from build123d import *

# Parameters (mm, degrees)
F0_R     = 0.6
F1_DEPTH = 1.7
F3_DEPTH = 2
F5_DEPTH = 1
F6_R     = 1.1
F7_DEPTH = 2.701
F8_R     = 2.35
F8_R_2   = 1.1
F9_DEPTH = 2


with BuildPart() as f1:
    # F0 (on Top) → F1 (new body)
    with BuildSketch(Plane.XY):
        with BuildLine():
            ThreePointArc((2.2299103121, -2.5), (3.057180036, -1.369726333), (3.35, 0))
            ThreePointArc((3.35, 0), (3.057180036, 1.369726333), (2.2299103121, 2.5))
            ThreePointArc((2.2299103121, 2.5), (0, 3.35), (-2.2299103121, 2.5))
            ThreePointArc((-2.2299103121, 2.5), (-3.35, 0), (-2.2299103121, -2.5))
            ThreePointArc((-2.2299103121, -2.5), (0, -3.35), (2.2299103121, -2.5))
        make_face()
        with BuildLine():
            ThreePointArc((2.2299103121, 2.5), (3.057180036, 1.369726333), (3.35, 0))
            ThreePointArc((3.35, 0), (3.057180036, -1.369726333), (2.2299103121, -2.5))
            Line((2.2299103121, -2.5), (14, -2))
            ThreePointArc((14, -2), (16, 0), (14, 2))
            Line((14, 2), (2.2299103121, 2.5))
        make_face()
        with Locations((4, 0)):
            Circle(F0_R, mode=Mode.SUBTRACT)
        with Locations((6, 0)):
            Circle(F0_R, mode=Mode.SUBTRACT)
        with Locations((8, 0)):
            Circle(F0_R, mode=Mode.SUBTRACT)
        with Locations((10, 0)):
            Circle(F0_R, mode=Mode.SUBTRACT)
        with Locations((12, 0)):
            Circle(F0_R, mode=Mode.SUBTRACT)
        with Locations((14, 0)):
            Circle(F0_R, mode=Mode.SUBTRACT)
        with BuildLine():
            ThreePointArc((-2.2299103121, -2.5), (-3.35, 0), (-2.2299103121, 2.5))
            Line((-2.2299103121, 2.5), (-9.1662129992, 2.2053419782))
            Line((-9.1662129992, 2.2053419782), (-9.1662129992, -2.2053419782))
            Line((-9.1662129992, -2.2053419782), (-2.2299103121, -2.5))
        make_face()
        with Locations((-8, 0)):
            Circle(F0_R, mode=Mode.SUBTRACT)
        with Locations((-6, 0)):
            Circle(F0_R, mode=Mode.SUBTRACT)
        with Locations((-4, 0)):
            Circle(F0_R, mode=Mode.SUBTRACT)
    extrude(amount=F1_DEPTH)

    # F2 (on face) → F3 (join)
    with BuildSketch(Plane.XY.offset(1.7)):
        with BuildLine():
            ThreePointArc((2.2299103121, -2.5), (3.057180036, -1.369726333), (3.35, 0))
            ThreePointArc((3.35, 0), (3.057180036, 1.369726333), (2.2299103121, 2.5))
            ThreePointArc((2.2299103121, 2.5), (0, 3.35), (-2.2299103121, 2.5))
            ThreePointArc((-2.2299103121, 2.5), (-3.35, 0), (-2.2299103121, -2.5))
            ThreePointArc((-2.2299103121, -2.5), (0, -3.35), (2.2299103121, -2.5))
        make_face()
    extrude(amount=F3_DEPTH)

    # F4 (on face) → F5 (cut)
    with BuildSketch(Plane(origin=(0, 0, 0), x_dir=(1, 0, 0), z_dir=(0, 0, -1))):
        with BuildLine():
            ThreePointArc((1.5642654428, 1.7537313433), (-2.35, 0), (1.5642654428, -1.7537313433))
            ThreePointArc((1.5642654428, -1.7537313433), (2.35, 0), (1.5642654428, 1.7537313433))
        make_face()
    extrude(amount=-F5_DEPTH, mode=Mode.SUBTRACT)

    # F6 (on face) → F7 (cut, through all)
    with BuildSketch(Plane(origin=(0, 0, 1), x_dir=(1, 0, 0), z_dir=(0, 0, -1))):
        Circle(F6_R)
    extrude(amount=-F7_DEPTH, mode=Mode.SUBTRACT)

    # F8 (on face) → F9 (cut, through all)
    with BuildSketch(Plane.XY.offset(3.7)):
        Circle(F8_R)
        Circle(F8_R_2, mode=Mode.SUBTRACT)
    extrude(amount=-F9_DEPTH, mode=Mode.SUBTRACT)


solid = f1.part
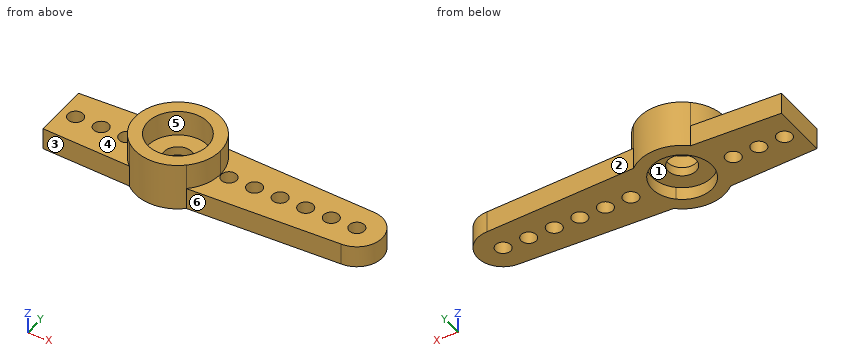
CAD build for the part. Positions are in the model's coordinates, mm. Face numbers are marked on the shaded views. A direction names the side the tool comes from. Give positions to 0.01 mm unless a question says otherwise; leave off trailing zeros. Loops run counter-clockwise (first coordinate to the right, second up) from the corner with the lowest first, then second, coordinate; pieces in that order, holes last. Notation, with made-up numbers: M -28.5,-17.5 L 28.5,-17.5 A36 ccw 28.5,20.5 Z; hole C 67,1.5 d11. An arc over 180 degrees is marked long. Answer in a Markdown table with one row per item. Add a question column.
Item 1: Band-saw the part on A-A on z = 1.4. Give the number of separate pieces and of enclosed holes in the cut face, then the cut area to 3 significant figures.
Item 2: Probe probe 1 along Y at (x, z) = (0, 3.1); probe 2 along Y at (x, z) = (14, 1.3); probe 3 along X at (y, z) = (-2, 2.6). List the from-to ranges inside material, lowest first.
Item 3: Band-saw the part on C-C on z = 3. Give the cut face in (x, y), then the cut area to 3 significant figures.
Item 4: Mould opens along X. For the marked faces 1, 2, 3 and 4 say: +X half, -X half, draft (parallel to the pull), parting line (faces both ways), or undercut.
Item 5: Band-saw the part on D-D on y = -1.5. Give the cut face in (x, z), then the cut area to 3 significant figures.
Item 6: Drop flat-ended pins along their axis: P1, Ø2.5, axis at x = 0, y = 0, coming from the -Z side; P2, Ø0.7, axis at x = 14, y = 0, coming from the -Z side; P3, Ø2, axis at y = -2, z = 2, coming from the -X side; P4, Ø1.4, axis at x = 12, y = 0, coming from the +Z side. Give the stop position or say it passes through.
Item 7: Band-saw the part on B-B on x = 8. Give the cut face in (y, z), then the cut area to 3 significant figures.
Item 8: Tool access for the marked faces 5 and 6: list every direction of +Z, -Z, +X, -X, +Y, -Y with a clear straight run to the whole face (end or side of a thin tool).
Reply:
| question | item | result |
|---|---|---|
| 1 | separate pieces | 1 |
| 1 | enclosed holes | 10 |
| 1 | area | 105 mm^2 |
| 2 | probe 1 | y = -3.35 to -2.35, 2.35 to 3.35 |
| 2 | probe 2 | y = -2 to -0.6, 0.6 to 2 |
| 2 | probe 3 | x = -2.69 to -1.23, 1.23 to 2.69 |
| 3 | outline | C 0,0 d6.7; hole C 0,0 d4.7 |
| 3 | area | 17.9 mm^2 |
| 4 | face 1 | undercut |
| 4 | face 2 | +X half |
| 4 | face 3 | -X half |
| 4 | face 4 | draft |
| 5 | outline | M -9.17,0 L -1.81,0 L -1.81,1 L 1.81,1 L 1.81,0 L 15.32,0 L 15.32,1.7 L 3,1.7 L 3,3.7 L 1.81,3.7 L 1.81,1.7 L -1.81,1.7 L -1.81,3.7 L -3,3.7 L -3,1.7 L -9.17,1.7 Z |
| 5 | area | 42.8 mm^2 |
| 6 | P1 | stops at z = 1 |
| 6 | P2 | passes through |
| 6 | P3 | stops at x = -9.17 |
| 6 | P4 | stops at z = 1.7 |
| 7 | outline | M -2.25,0 L -0.6,0 L -0.6,1.7 L -2.25,1.7 Z; M 0.6,0 L 2.25,0 L 2.25,1.7 L 0.6,1.7 Z |
| 7 | area | 5.63 mm^2 |
| 8 | face 5 | +Z |
| 8 | face 6 | +Z, -Z, +X, -Y |
